```python
from build123d import *

# Parameters (mm, degrees)
BOSS_EXTRUDE1_DEPTH = 2.54
SKETCH2_R           = 3.175
CUT_EXTRUDE1_DEPTH  = 116.115535007
CUT_EXTRUDE2_DEPTH  = 116.115535007
SKETCH4_R           = 3.175
BOSS_EXTRUDE2_DEPTH = 8.89
SKETCH5_R           = 4.445
BOSS_EXTRUDE3_DEPTH = 2.54


with BuildPart() as part:
    # Sketch1 → Boss-Extrude1 (new, symmetric)
    with BuildSketch(Plane.XY):
        with BuildLine():
            Line((-101.6, 12.7), (101.6, 12.7))
            ThreePointArc((101.6, 12.7), (114.3, 0), (101.6, -12.7))
            Line((101.6, -12.7), (-101.6, -12.7))
            ThreePointArc((-101.6, -12.7), (-114.3, 0), (-101.6, 12.7))
        make_face()
    extrude(amount=BOSS_EXTRUDE1_DEPTH, both=True)

    # Sketch2 → Cut-Extrude1 (cut, through all)
    with BuildSketch(Plane.XY.offset(2.54)):
        with Locations((101.6, 0)):
            Circle(SKETCH2_R)
    extrude(amount=-CUT_EXTRUDE1_DEPTH, mode=Mode.SUBTRACT)

    # Sketch3 → Cut-Extrude2 (cut, through all)
    with BuildSketch(Plane.XY.offset(2.54)):
        with BuildLine():
            Line((-46.228, 4.572), (45.72, 4.572))
            ThreePointArc((45.72, 4.572), (50.292, 0), (45.72, -4.572))
            Line((45.72, -4.572), (-46.228, -4.572))
            ThreePointArc((-46.228, -4.572), (-50.8, 0), (-46.228, 4.572))
        make_face()
    extrude(amount=-CUT_EXTRUDE2_DEPTH, mode=Mode.SUBTRACT)

    # Sketch4 → Boss-Extrude2 (add)
    with BuildSketch(Plane.XY.offset(2.54)):
        with Locations((-101.6, 0)):
            Circle(SKETCH4_R)
    extrude(amount=BOSS_EXTRUDE2_DEPTH)

    # Sketch5 → Boss-Extrude3 (add)
    with BuildSketch(Plane.XY.offset(11.43)):
        with Locations((-101.6, 0)):
            Circle(SKETCH5_R)
    extrude(amount=-BOSS_EXTRUDE3_DEPTH)


solid = part.part
```
Could you check a few things on this model? Use its own coordinates, in mm. A direction names the side the tool comes from. Coordinates: 2 decimals unless noted, no trailing zeros. Write each loop counter-clockwise with the first axis right and the second up, starting at its lowest first coordinate (ties: lowest second). Pieces come first, ordered by that corner, then holes. Notation, with made-up numbers: M 57.5,16 L 74.5,16 A17 ccw 74.5,28 Z; hole C 11,50.5 d11. An arc over 180 degrees is marked long. Answer as CSV lines item,"result". Start each with the question number.
1) Please list where these lines run through material, in increasing order: line 1 (Y direction, x = 101.6, z = 1.3) (3 decimals); line 2 (Z direction, x = 72, y = -11); line 3 (X direction, y = -8.75, z = 2). Write a range as from..to.
2) For faces 4 (the cylindrical face through (-104.77, 0.14, 5.67)), 5 (the flat face through (-1, 4.572, 0)), 6 (the cylindrical face through (-97.494, -1.702, 10.178)), 7 (the flat face through (-1, 12.7, 0)), which set-ups out of +Z, -Z, +X, -X, +Y, -Y let a thin tool reach every point of the face, with its end or its side?
3) For P1, Ø4, axis at x = -34.5, y = -1.5, coming from the -Z side; P2, Ø10, axis at x = 7.5, y = -5.5, coming from the +Z side, each with a flat end and sliding along its axis, tell me the tip position at first contact or that it passes through.
4) I want a section at B-B, the plane z = 0.25. Please give me the cut outline in (x, y) (3 decimals).
5) I want a section at D-D, the plane x = 73. Please give me the cut outline in (y, z), and give its area (3 significant figures).
6) I want a section at A-A, the plane x = -19. Please give me the cut outline in (y, z), and give its area (3 significant figures).
7) I want a section at C-C, the plane y = 0. Please give me the cut outline in (x, z) (3 decimals).
8) We'd pull the mould along Z, two halves only. Please class faces 1 (the cylindrical face through (114.297, 0.279, 0.036)), 2 (the flat face through (-102, 0, 11.43)), 3 (the flat face through (-105, 1, 8.89)): +Z half, -Z half, draft (parallel to the pull), parting line (faces both ways), or undercut.
Data:
1,line 1,"y = -12.7..-3.175, 3.175..12.7"
1,line 2,"z = -2.54..2.54"
1,line 3,"x = -110.8..110.8"
2,face 4,"none"
2,face 5,"+Z, -Z"
2,face 6,"+Z"
2,face 7,"+Z, -Z, +X, -X, +Y"
3,P1,"passes through"
3,P2,"stops at z = 2.54"
4,outline,"M -101.6,-12.7 L 101.6,-12.7 A12.7 ccw 101.6,12.7 L -101.6,12.7 A12.7 ccw Z; hole M -46.228,-4.572 L 45.72,-4.572 A4.572 ccw 45.72,4.572 L -46.228,4.572 A4.572 ccw Z; hole C 101.6,0 d6.35"
5,outline,"M -12.7,-2.54 L 12.7,-2.54 L 12.7,2.54 L -12.7,2.54 Z"
5,area,"129 mm^2"
6,outline,"M -12.7,-2.54 L -4.57,-2.54 L -4.57,2.54 L -12.7,2.54 Z; M 4.57,-2.54 L 12.7,-2.54 L 12.7,2.54 L 4.57,2.54 Z"
6,area,"82.6 mm^2"
7,outline,"M -114.3,-2.54 L -50.8,-2.54 L -50.8,2.54 L -98.425,2.54 L -98.425,8.89 L -97.155,8.89 L -97.155,11.43 L -106.045,11.43 L -106.045,8.89 L -104.775,8.89 L -104.775,2.54 L -114.3,2.54 Z; M 50.292,-2.54 L 98.425,-2.54 L 98.425,2.54 L 50.292,2.54 Z; M 104.775,-2.54 L 114.3,-2.54 L 114.3,2.54 L 104.775,2.54 Z"
8,face 1,"draft"
8,face 2,"+Z half"
8,face 3,"undercut"
